Here's how the part is built. I have some questions about the finished solid (model axes, mm). Face numbers are marked on the shaded views. A direction names the side the tool comes from. Coordinates: 2 decimals unless noted, no trailing zeros. Write each loop counter-clockwise with the first axis right and the second up, starting at its lowest first coordinate (ties: lowest second). Pieces come first, ordered by that corner, then holes. Notation, with made-up numbers: (5.5, 64) - (30.5, 64) arc R9 ccw to (30.5, 79) - close; hole circle Ø3 at (54.5, -13). An arc over 180 degrees is marked (long way). Answer in a Markdown table with one row per item. Add a question column.
Item 1: Imagine slicing it at B-B (y = -107). Please give me the cut outline in (x, z).
Item 2: I'm going to push flat-ended pins straight in: pin 1 (5 mm diameter, centred on x = 7.5, y = -125, fed in from -Z); pin 2 (5 mm diameter, centred on x = 6.5, y = -155.5, fed in from +Z); pin 3 (8 mm diameter, centred on x = 11, y = -173.5, fed in from -Z). Where does each tip first touch, or does it pass through?
Item 3: Imagine slicing it at A-A (x = 0). Please give me the cut outline in (y, z), plus the area to 3 significant figures.
Item 4: If I drill on probe 1 along Y at (x, z) = (0, 68); probe 2 along X at (y, z) = (-213, 59); probe 3 along Y at (x, z) = (-4.5, 45.5), over which ranges is the centre line in solid material (lowest first)? Write a range as from..to.
Item 5: Which directions (+Z, -Z, +X, -X, +Y, -Y) give clear straight access to the entire face, cutting with the end or side of a thin tool? Please do the marked faces 4 and 5.
Item 6: We'd pull the mould along Y, two halves only. Please class the marked faces 1, 2 and 3: +Y half, -Y half, draft (parallel to the pull), parting line (faces both ways), or undercut.
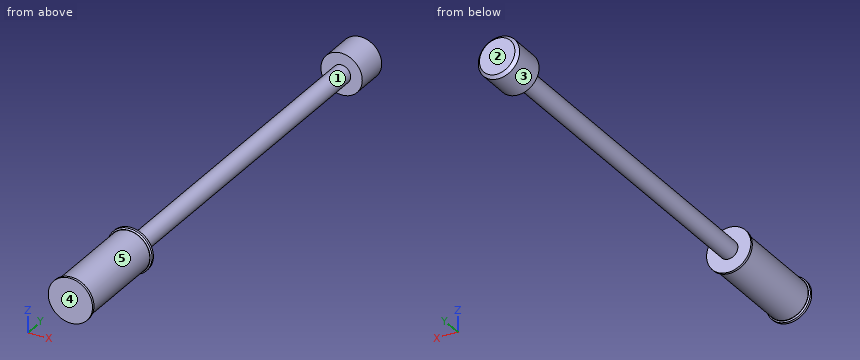
from build123d import *

# Parameters (mm, degrees)
SKETCH016_R     = 7.75
PAD006_DEPTH    = 300
SKETCH017_R     = 17.5
PAD007_DEPTH    = 30
CHAMFER006_SIZE = 2.5
SKETCH018_R     = 17.5
PAD008_DEPTH    = 80
SKETCH019_R     = 18.75
PAD009_DEPTH    = 3
SKETCH020_R     = 18.75
PAD010_DEPTH    = 3
CHAMFER007_SIZE = 1


with BuildPart() as part:
    # Sketch016 → Pad006 (new body)
    with BuildSketch(Plane.XZ):
        with Locations((0, 60.015743)):
            Circle(SKETCH016_R)
    extrude(amount=PAD006_DEPTH)

    # Sketch017 (on Face2 of Pad006) → Pad007 (join)
    with BuildSketch(Plane(origin=(0, 0, 0), x_dir=(1, 0, 0), z_dir=(0, 1, 0))):
        with Locations((0, -60.094143)):
            Circle(SKETCH017_R)
    extrude(amount=PAD007_DEPTH)

    # Chamfer006
    chamfer006_edges = [part.edges().sort_by_distance(p)[0] for p in [
        (-17.5, 30, 60.094143),
    ]]
    chamfer(chamfer006_edges, length=CHAMFER006_SIZE)

    # Sketch018 (on Face6 of Chamfer006) → Pad008 (join)
    with BuildSketch(Plane.XZ.offset(300)):
        with Locations((0, 60.040283)):
            Circle(SKETCH018_R)
    extrude(amount=PAD008_DEPTH)

    # Sketch019 (on Face8 of Pad008) → Pad009 (join)
    with BuildSketch(Plane.XZ.offset(380)):
        with Locations((0, 60.03339)):
            Circle(SKETCH019_R)
    extrude(amount=PAD009_DEPTH)

    # Sketch020 (on Face6 of Pad009) → Pad010 (join)
    with BuildSketch(Plane(origin=(0, -300, 0), x_dir=(1, 0, 0), z_dir=(0, 1, 0))):
        with Locations((0, -60.018958)):
            Circle(SKETCH020_R)
    extrude(amount=PAD010_DEPTH)

    # Chamfer007
    chamfer007_edges = [part.edges().sort_by_distance(p)[0] for p in [
        (-18.75, -300, 60.018958),
        (-18.75, -380, 60.03339),
    ]]
    chamfer(chamfer007_edges, length=CHAMFER007_SIZE)


solid = part.part
Here are the results:
| question | item | result |
|---|---|---|
| 1 | outline | circle Ø15.5 at (0, 60.02) |
| 2 | pin 1 | stops at z = 54.09 |
| 2 | pin 2 | stops at z = 66.65 |
| 2 | pin 3 | stops at z = 56.69 |
| 3 | outline | (-383, 41.28) - (-381, 41.28) - (-380, 42.28) - (-380, 42.54) - (-300, 42.54) - (-300, 42.27) - (-299, 41.27) - (-297, 41.27) - (-297, 52.27) - (0, 52.27) - (0, 42.59) - (27.5, 42.59) - (30, 45.09) - (30, 75.09) - (27.5, 77.59) - (0, 77.59) - (0, 67.77) - (-297, 67.77) - (-297, 78.77) - (-299, 78.77) - (-300, 77.77) - (-300, 77.54) - (-380, 77.54) - (-380, 77.78) - (-381, 78.78) - (-383, 78.78) - close |
| 3 | area | 8,670 mm2 |
| 4 | probe 1 | y = -383..-297, 0..30 |
| 4 | probe 2 | x = -7.68..7.68 |
| 4 | probe 3 | y = -383..-297, 0..29.73 |
| 5 | face 4 | +Z, -Z, +X, -X, -Y |
| 5 | face 5 | none |
| 6 | face 1 | undercut |
| 6 | face 2 | +Y half |
| 6 | face 3 | draft |
